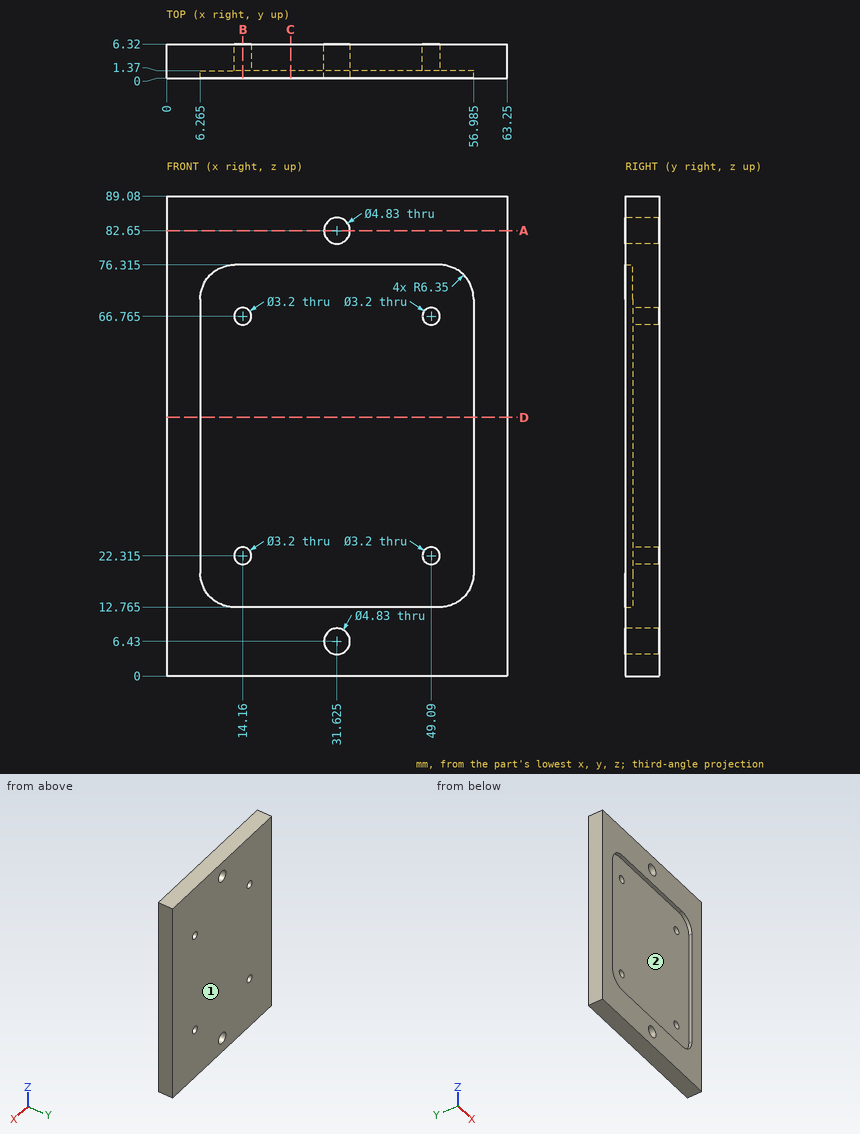
Geometry check sheet. Reference: drawing and pictorial views, mm from the part's lowest x, y, z. Coordinates: 2 decimals unless noted, no trailing zeros. Loops run counter-clockwise (first coordinate to the right, second up) from the corner with the lowest first, then second, coordinate; pieces in that order, holes last.
1) Sectioned sample at B-B (x = 14.16). Record the boundary of the cut face in (y, z) (3 decimals).
2) Release check for a two-part mould opening along X. For the marked faces 1 and 2 record: released by +X, released by -X, zero draft, split by the parting line, or undercut.
3) Sectioned sample at D-D (z = 48). Record the boundary of the cut face in (x, y) (3 decimals), and give its area (3 significant figures).
4) Sectioned sample at A-A (z = 82.65). Record the boundary of the cut face in (x, y), and give its area (3 significant figures).
5) Gauge pin test, flat ends, axial feed: pin 1 (10 mm diameter, centred on x = 19.5, z = 22.5, fed in from -Y); pin 2 (4.5 mm diameter, centred on x = 31.625, z = 82.65, fed in from -Y) (1 decimal). Record the tip position at first contact, or that the pin passes through.
6) Material ranges on probe 1 along Z at (x, y) = (14.16, 3.45) (3 decimals); probe 2 along X at (y, z) = (0.75, 54) (3 decimals); probe 3 along Y at (x, z) = (30, 45), recorded low to high.
7) Sectioned sample at C-C (x = 23). Record the boundary of the cut face in (y, z) (3 decimals).
Check sheet entries:
1. outline: (0, 0) - (6.32, 0) - (6.32, 20.715) - (1.37, 20.715) - (1.37, 12.765) - (0, 12.765) - close; (0, 76.315) - (1.37, 76.315) - (1.37, 68.365) - (6.32, 68.365) - (6.32, 89.08) - (0, 89.08) - close; (1.37, 23.915) - (6.32, 23.915) - (6.32, 65.165) - (1.37, 65.165) - close
2. face 1: zero draft
2. face 2: undercut
3. outline: (0, 0) - (6.265, 0) - (6.265, 1.37) - (56.985, 1.37) - (56.985, 0) - (63.25, 0) - (63.25, 6.32) - (0, 6.32) - close
3. area: 330 mm2
4. outline: (0, 0) - (29.21, 0) - (29.21, 6.32) - (0, 6.32) - close; (34.04, 0) - (63.25, 0) - (63.25, 6.32) - (34.04, 6.32) - close
4. area: 369 mm2
5. pin 1: stops at y = 1.37
5. pin 2: passes through
6. probe 1: z = 0 to 20.715, 23.915 to 65.165, 68.365 to 89.08
6. probe 2: x = 0 to 6.265, 56.985 to 63.25
6. probe 3: y = 1.37 to 6.32
7. outline: (0, 0) - (6.32, 0) - (6.32, 89.08) - (0, 89.08) - (0, 76.315) - (1.37, 76.315) - (1.37, 12.765) - (0, 12.765) - close
